Verification items for the finished model (mm, model axes). Face numbers are marked on the shaded views. A direction names the side the tool comes from. Give positions to 0.01 mm unless a question says otherwise; leave off trailing zeros. One line per item, written item: value. Start each with the question number.
1. Mould release check, pull along Y, two halves, no side actions. Record for the marked faces 1, 2, 3 and 4: pulls with the +Y half, pulls with the -Y half, needs draft (parallel to the pull), parting line crosses it, or undercut.
2. Gauge pin test, flat ends, axial feed: pin 1 (7 mm diameter, centred on x = 0, z = 0, fed in from -Y); pin 2 (1.6 mm diameter, centred on y = 2.5, z = 0, fed in from -X); pin 3 (2 mm diameter, centred on x = 5.5, y = 4, fed in from -Z); pin 4 (1 mm diameter, centred on y = 4.5, z = 7.5, fed in from -X). Record the tip position at first contact, or that the pin passes through.
3. Sectioned sample at A-A (x = 0). Count the separate pieces of the cut face and the enclosed holes in it, plus the area to 3 significant figures.
4. Access from +Z, -Z, +X, -X, +Y, -Y to the whole of each face (thin tool, end or side, straight path). Record for the marked faces 5 and 6.
5. Scan lines: L1, parallel to Y at x = 8.5, z = -9.5; L2, parallel to X at y = 4.65, z = 0; L3, parallel to X at y = 3.95, z = 0. Record each from-to range of solid material in increasing order. Write a range as [from, to].
from build123d import *

# Parameters (mm, degrees)
SKETCH1_R           = 13.25
BOSS_EXTRUDE1_DEPTH = 5
SKETCH5_R           = 0.5
CUT_EXTRUDE1_DEPTH  = 5


with BuildPart() as part:
    # Sketch1 → Boss-Extrude1 (new body)
    with BuildSketch(Plane(origin=(0, 0, 0), x_dir=(1, 0, 0), z_dir=(0, 1, 0))):
        with Locations(Location((0, 0, 0), (0, 0, 270))):
            Circle(SKETCH1_R)
        with BuildLine():
            Line((2.25, 1.58113883), (2.25, -1.58113883))
            ThreePointArc((2.25, -1.58113883), (-2.75, 0), (2.25, 1.58113883))
        make_face(mode=Mode.SUBTRACT)
    extrude(amount=BOSS_EXTRUDE1_DEPTH)

    # Sketch4 → Cut-Revolve1 (revolve, cut)
    with BuildSketch(Plane.ZY):
        Polygon((12.75, 4.5), (10.75, 2.5), (12.75, 0.5), (13.25, 0.5), (13.25, 4.5), align=None)
    revolve(axis=Axis((0, 5, 0), (0, -1, 0)), mode=Mode.SUBTRACT)

    # Sketch5 → Cut-Extrude1 (cut)
    with BuildSketch(Plane(origin=(0, 5, 0), x_dir=(1, 0, 0), z_dir=(0, 1, 0))):
        with Locations(Location((-12, 0, 0), (0, 0, 270))):
            Circle(SKETCH5_R)
        with Locations(Location((12, 0, 0), (0, 0, 143.030391189))):
            Circle(SKETCH5_R)
        with Locations(Location((0, 12, 0), (0, 0, 270))):
            Circle(SKETCH5_R)
        with Locations(Location((0, -12, 0), (0, 0, 270.000003371))):
            Circle(SKETCH5_R)
    extrude(amount=-CUT_EXTRUDE1_DEPTH, mode=Mode.SUBTRACT)


solid = part.part
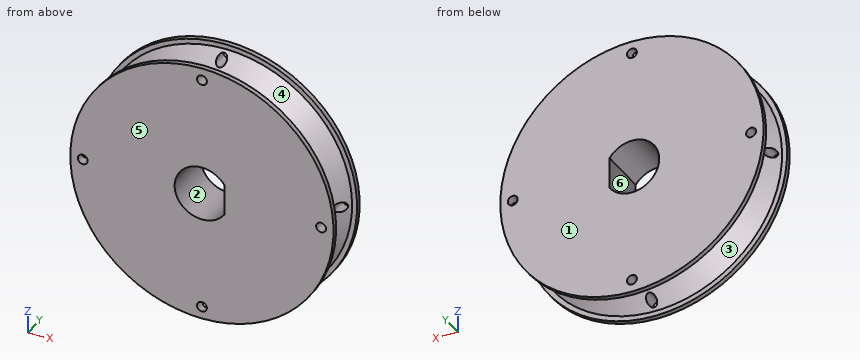
Results are:
1. face 1: pulls with the +Y half
1. face 2: needs draft
1. face 3: undercut
1. face 4: undercut
2. pin 1: stops at y = 0
2. pin 2: stops at x = -11.53
2. pin 3: stops at z = -12.41
2. pin 4: stops at x = -11.25
3. separate pieces: 6
3. enclosed holes: 0
3. area: 88.0 mm^2
4. face 5: +Z, -Z, +X, -X, -Y
4. face 6: +Y, -Y
5. L1: y = [0, 0.5], [4.5, 5]
5. L2: x = [-13.25, -12.5], [-11.5, -2.75], [2.25, 11.5], [12.5, 13.25]
5. L3: x = [-11.5, -2.75], [2.25, 11.5]
